Autodesk Inventor part; units mm, degrees
ref_plane "YZ Plane" through (0, 0, 0) normal (1, 0, 0) x (0, 1, 0)
ref_plane "XZ Plane" through (0, 0, 0) normal (0, 1, 0) x (-1, 0, 0)
ref_plane "XY Plane" through (0, 0, 0) normal (0, 0, 1) x (1, 0, 0)
sketch "Sketch1" plane through (0, 0, 0) normal (0, 1, 0) x (-1, 0, 0)
  circle A0 centre (0, 0) radius 2.6
  circle A1 centre (0, 0) radius 7.3625 construction
  circle A2 centre (0, 46) radius 2.6
  circle A3 centre (0, 46) radius 7.3625 construction
  line L0 (7.3625, 0) -> (7.3625, 46)
  line L1 (-7.3625, 46) -> (-7.3625, 0)
  arc A4 (-7.3625, 0) -> (7.3625, 0) centre (0, 0) ccw
  arc A5 (7.3625, 46) -> (-7.3625, 46) centre (0, 46) ccw
  dimension "d0" = 5.2
  dimension "d1" = 4.7625
  dimension "d2" = 46
extrude "Extrusion1" add sketch "Sketch1" along normal blind 5
properties part number "CNC-019-ZAxisBallScrewStabilizerShim2" material "ABS Plastic"
The listing builds one solid part. Answer for the finished solid, in the listing's coordinates (mm). Coordinates: 2 decimals unless noted, no trailing zeros. Write each loop counter-clockwise with the first axis right and the second up, starting at its lowest first coordinate (ties: lowest second). Pieces come first, ordered by that corner, then holes. Notation, with made-up numbers: (70, -7) - (95, -7) arc R7 ccw to (95, 0) - close; hole circle Ø4 at (50.25, 39). An arc over 180 degrees is marked (long way). Return JSON: item names as keys, results as strings. Group by question number.
Q1. Find the intervals of material crossed by line 1 along Z through (x, y) = (0, 2.05); line 2 along Z through (x, y) = (-1.5, 1); line 3 along Z through (x, y) = (5.5, 0.75), in increasing order. Write a range as [from, to].
Q2. The part is cut by section A-A on x = 0. Write down the section's boundary in (y, z).
Q3. A flat-ended cylindrical pin translates along its axis: pin 1 Ø2 at (x, y) = (-5, 3.5) entering from -Z. Find the tip coordinate at first contact, or state that the pin passes through.
Q4. For a pull along X with two mould halves and no side action, classify faces 1 (the cylindrical face through (0.56, 2.46, 48.54)), 2 (the flat face through (-7.362, 2, 23)), 3 (the cylindrical face through (0.338, 2.465, -2.578)), 4 (the flat face through (7.362, 2, 23)) as +X half, -X half, draft (parallel to the pull), parting line (faces both ways), or undercut.
Q5. The part is cut by section B-B on y = 1.5. Write down the section's boundary in (x, z) (1 decimal).
Q6. The part is cut by section D-D on z = -1. Write down the section's boundary in (x, y), and give its area (3 significant figures).
Q7. The part is cut by section C-C on z = 48. Write down the section's boundary in (x, y), and give its area (3 significant figures).
Evaluation:
{
 "1": {"line 1": "z = [-7.36, -2.6], [2.6, 43.4], [48.6, 53.36]", "line 2": "z = [-7.21, -2.12], [2.12, 43.88], [48.12, 53.21]", "line 3": "z = [-4.89, 50.89]"},
 "2": {"outline": "(0, -7.36) - (5, -7.36) - (5, -2.6) - (0, -2.6) - close; (0, 2.6) - (5, 2.6) - (5, 43.4) - (0, 43.4) - close; (0, 48.6) - (5, 48.6) - (5, 53.36) - (0, 53.36) - close"},
 "3": {"pin 1": "stops at z = -6.18"},
 "4": {"face 1": "undercut", "face 2": "-X half", "face 3": "undercut", "face 4": "+X half"},
 "5": {"outline": "(-7.4, 0) arc R7.4 ccw to (7.4, 0) - (7.4, 46) arc R7.4 ccw to (-7.4, 46) - close; hole circle Ø5.2 at (0, 0); hole circle Ø5.2 at (0, 46)"},
 "6": {"outline": "(-7.29, 0) - (-2.4, 0) - (-2.4, 5) - (-7.29, 5) - close; (2.4, 0) - (7.29, 0) - (7.29, 5) - (2.4, 5) - close", "area": "48.9 mm2"},
 "7": {"outline": "(-7.09, 0) - (-1.66, 0) - (-1.66, 5) - (-7.09, 5) - close; (1.66, 0) - (7.09, 0) - (7.09, 5) - (1.66, 5) - close", "area": "54.2 mm2"}
}
